Part model, mm, in its own coordinate system. A direction names the side the tool comes from. Coordinates: 2 decimals unless noted, no trailing zeros. Loops run counter-clockwise (first coordinate to the right, second up) from the corner with the lowest first, then second, coordinate; pieces in that order, holes last. Notation, with made-up numbers: M -31,-28.75 L 21,-28.75 A14 cw 21,-3.75 Z; hole C 78.5,21.25 d8. An arc over 180 degrees is marked long. Use a Markdown table: item, result. Add a question column.
1) Pin check, flat tips, straight feed: pin 1 Ø4 at (x, y) = (-67, 47) entering from -Z; pin 2 Ø3 at (y, z) = (60.5, -55) entering from -X; pin 3 Ø10 at (y, z) = (66.5, -24) entering from -X. Stop position of each tip, or through.
2) Band-saw the part on A-A (z = 0). List the corners of the cut face in (x, y), plus the area to 3 significant figures.
3) Pull direction Z, two halves, no side cores. Call faces 1 (the flat face through (1, 4, -1)), 2 (the cylindrical face through (51.721, 104.958, 67.453)), 3 (the flat face through (1, 0, -1)), 4 (the cylindrical face through (-45.636, 56.258, -59.517)): released by +Z, released by -Z, zero draft, split by the parting line, or undercut.
4) Band-saw the part on C-C (y = 43.5). List the corners of the cut face in (x, z), plus the area to 3 significant figures.
5) Band-saw the part on B-B (x = 0). List the corners of the cut face in (y, z), plus the area to 3 significant figures.
6) Wall check: probe 1 along X at (y, z) = (34.5, 0); probe 2 along Y at (x, z) = (7, -30.5); probe 3 along X at (y, z) = (41.5, -41.5). Give the ranges that are in metal, low to high. Write a range as from..to.
7) Tool access for faces 5 (the flat face through (43, 110, -62)), 6 (the cylindrical face through (23.73, 49.3, 75.35)): list every direction of +Z, -Z, +X, -X, +Y, -Y with a clear straight run to the whole face (end or side of a thin tool).
from build123d import *

# Parameters (mm, degrees)
SKETCH1_R           = 79
BOSS_EXTRUDE1_DEPTH = 110
SHELL1_T            = -4


with BuildPart() as part:
    # Sketch1 → Boss-Extrude1 (new body)
    with BuildSketch(Plane(origin=(0, 0, 0), x_dir=(1, 0, 0), z_dir=(0, 1, 0))):
        with Locations(Location((0, 0, 0), (0, 0, 270))):
            Circle(SKETCH1_R)
    extrude(amount=BOSS_EXTRUDE1_DEPTH)

    # Shell1
    shell1_openings = [part.faces().sort_by_distance(p)[0] for p in [
        (0, 110, 0),
    ]]
    offset(amount=SHELL1_T, openings=shell1_openings, kind=Kind.INTERSECTION)

    # Sketch2 → Revolve1 (revolve)
    with BuildSketch(Plane(origin=(0, 0, 0), x_dir=(0, 0, -1), z_dir=(1, 0, 0))):
        with BuildLine():
            Line((79, 110), (83, 110))
            ThreePointArc((83, 110), (84.414213562, 109.414213562), (85, 108))
            Line((85, 108), (85, 102))
            ThreePointArc((85, 102), (84.414213562, 100.585786438), (83, 100))
            Line((83, 100), (79, 100))
            Line((79, 100), (79, 110))
        make_face()
    revolve(axis=Axis((0, -5.5, 0), (0, 1, 0)))


solid = part.part
Entries:
| question | item | result |
|---|---|---|
| 1 | pin 1 | z = -44.9 |
| 1 | pin 2 | x = -58.13 |
| 1 | pin 3 | x = -76.68 |
| 2 | outline | M -85,102 A2 ccw -83,100 L -79,100 L -79,0 L 79,0 L 79,100 L 83,100 A2 ccw 85,102 L 85,108 A2 ccw 83,110 L 75,110 L 75,4 L -75,4 L -75,110 L -83,110 A2 ccw -85,108 Z |
| 2 | area | 1,600 mm2 |
| 3 | face 1 | undercut |
| 3 | face 2 | split by the parting line |
| 3 | face 3 | zero draft |
| 3 | face 4 | undercut |
| 4 | outline | C 0,0 d158; hole C 0,0 d150 |
| 4 | area | 1,940 mm2 |
| 5 | outline | M 0,-79 L 100,-79 L 100,-83 A2 ccw 102,-85 L 108,-85 A2 ccw 110,-83 L 110,-75 L 4,-75 L 4,75 L 110,75 L 110,83 A2 ccw 108,85 L 102,85 A2 ccw 100,83 L 100,79 L 0,79 Z |
| 5 | area | 1,600 mm2 |
| 6 | probe 1 | -79..-75, 75..79 |
| 6 | probe 2 | 0..4 |
| 6 | probe 3 | -67.22..-62.47, 62.47..67.22 |
| 7 | face 5 | +Z, -Z, +X, -X, +Y |
| 7 | face 6 | -Y |
